Autodesk Fusion 360 part; units mm, degrees
sketch "Sketch1" plane through (0, 0, 0) normal (0, 1, 0) x (1, 0, 0)
  line L0 (0, 0) -> (11, 0)
  line L1 (11, 0) -> (11, -16.3)
  line L2 (11, -16.3) -> (0, -16.3)
  line L3 (0, -16.3) -> (0, 0)
  line L4 (1.5, -14.8) -> (1.5, -1.5) construction
  line L5 (1.5, -1.5) -> (9.5, -1.5) construction
  line L6 (9.5, -1.5) -> (9.5, -14.8) construction
  line L7 (9.5, -14.8) -> (1.5, -14.8) construction
  circle A0 centre (5.5, -8.5) radius 1.5
  line L8 (5.5, -14.8) -> (5.5, -8.5) construction
  point P0 (1.5, -1.5)
  point P1 (9.5, -1.5)
  point P2 (9.5, -14.8)
  point P3 (1.5, -14.8)
  dimension "d1" = 16.3
  dimension "d2" = 11
  dimension "d3" = 1.5
  dimension "d4" = 6.3
  dimension "d5" = 3
extrude "Extrude1" add sketch "Sketch1" along normal blind 0.1
hole "Hole1" at (1.5, 0, 14.8) at (1.5, 0, 1.5) at (9.5, 0, 1.5) at (9.5, 0, 14.8) direction (0, 1, 0) diameter 1.7 depth 12 tip angle 118
fillet "Fillet1" radius 1.5 4 edges at (11, 0.05, 16.3) (0, 0.05, 16.3) (0, 0.05, 0) (11, 0.05, 0)
equation "d1 = 11.3 mm + 5 mm"
equation "d2 = 8 mm + 3 mm"
Can you work these out from the model? Positions are in its coordinate system, mm. Coordinates: 2 decimals unless noted, no trailing zeros. Write each loop counter-clockwise with the first axis right and the second up, starting at its lowest first coordinate (ties: lowest second). Pieces come first, ordered by that corner, then holes. Notation, with made-up numbers: (11, 40) - (40, 40) arc R22 cw to (40, 78) - close; hole circle Ø5 at (35, -17). An arc over 180 degrees is marked (long way). Return JSON: item names as keys, results as strings.
Q1. If we section it at B-B (x = 5.5): Please give me the cut outline in (y, z).
Computed values:
{"outline": "(0, 0) - (0.1, 0) - (0.1, 7) - (0, 7) - close; (0, 10) - (0.1, 10) - (0.1, 16.3) - (0, 16.3) - close"}
Q2. Please list where these lines run through material, in increasing order: L1, parallel to X at y = 0.05, z = 1.5; L2, parallel to Z at x = 1.5, y = 0.05; L3, parallel to Z at x = 6.75, y = 0.05. Write a range as from..to.
Computed values:
{"L1": "x = 0..0.65, 2.35..8.65, 10.35..11", "L2": "z = 0..0.65, 2.35..13.95, 15.65..16.3", "L3": "z = 0..7.67, 9.33..16.3"}
Q3. If we section it at A-A (z = 8.5): Please give me the cut outline in (x, y).
Computed values:
{"outline": "(0, 0) - (4, 0) - (4, 0.1) - (0, 0.1) - close; (7, 0) - (11, 0) - (11, 0.1) - (7, 0.1) - close"}
Q4. If we section it at D-D (y = 0.05): Please give me the cut outline in (x, z), then the cut area to 3 significant figures.
Computed values:
{"outline": "(0, 1.5) arc R1.5 ccw to (1.5, 0) - (9.5, 0) arc R1.5 ccw to (11, 1.5) - (11, 14.8) arc R1.5 ccw to (9.5, 16.3) - (1.5, 16.3) arc R1.5 ccw to (0, 14.8) - close; hole circle Ø1.7 at (1.5, 1.5); hole circle Ø1.7 at (1.5, 14.8); hole circle Ø3 at (5.5, 8.5); hole circle Ø1.7 at (9.5, 1.5); hole circle Ø1.7 at (9.5, 14.8)", "area": "161 mm2"}
Q5. If we section it at C-C (x = 9): Please give me the cut outline in (y, z), then the cut area to 3 significant figures.
Computed values:
{"outline": "(0, 0) - (0.1, 0) - (0.1, 0.81) - (0, 0.81) - close; (0, 2.19) - (0.1, 2.19) - (0.1, 14.11) - (0, 14.11) - close; (0, 15.49) - (0.1, 15.49) - (0.1, 16.3) - (0, 16.3) - close", "area": "1.36 mm2"}
Q6. I'm going to push a flat-ended pin straight in: pin 1 Ø5 at (x, z) = (5.5, 8.5) entering from +Y. Where does the tip first touch, or does it pass through?
Computed values:
{"pin 1": "stops at y = 0.1"}
